Read the model definition and answer for the solid it produces. Units are mm, in the model's axes. A direction names the side the tool comes from. Coordinates: 2 decimals unless noted, no trailing zeros. Order: outer loops, then holes, each group sorted by start corner. A loop starts at its lowest first (then second) coordinate and runs counter-clockwise, first axis right, second up. Notation, with made-up numbers: (16, 17.5) -> (52, 17.5) arc R22 cw to (52, 34.5) -> close; hole circle Ø4 at (74, 6). An arc over 180 degrees is marked (long way). Answer as a JSON object with one key per item and string values. Group by question number.
1) Determine the mould class of faces 1 (the cylindrical face through (-6.17, 1.48, 4.68)), 2 (the cylindrical face through (0.931, 7.93, 2.957)), 3 (the flat face through (1.1, 13, -3.1)), 4 (the cylindrical face through (1.352, 7.93, 4.292)) for opening direction X: released by +X, released by -X, zero draft, split by the parting line, or undercut.
2) Section C-C on x = 0 is taken. Determine the outline of the cut face in (y, z).
3) Given pin 1 (4 mm diameter, centred on x = 4.95, z = 4.95, fed in from +Y); pin 2 (1 mm diameter, centred on x = 2.5, y = 9, fed in from +Z); pin 3 (4 mm diameter, centred on x = 4.5, y = 6.5, fed in from +Z); pin 4 (2 mm diameter, centred on x = 4.95, z = -4.95, fed in from +Y), each flat-ended and moving along its own axis, determine where each tip first touches the part or whether it passes through.
4) Consider L1, parallel to X at y = 2.25, z = 4.5; L2, parallel to Z at x = -5, y = 0.5; L3, parallel to X at y = 1.5, z = 5.5. Determine where each line is inside the solid, lowest interval first.
5) Section B-B on y = 8 is taken. Determine the outline of the cut face in (x, z).
6) Section D-D on y = 4.5 is taken. Determine the outline of the cut face in (x, z).
7) Section A-A on z = 0 is taken. Determine the outline of the cut face in (x, y), and give its area (3 significant figures).
8) A tool of negligible diameter and unlimited length cuts with its end or side. For faces 5 (the cylindrical face through (3.57, 7.39, -1.48)), 6 (the flat face through (-5, 3, 0)), from which of +Z, -Z, +X, -X, +Y, -Y can it reach the whole face along a straight path? Write none if from no direction.
from build123d import *

# Parameters (mm, degrees)
CROQUIS1_R                 = 12.5
CROQUIS1_R_2               = 1.25
SALIENTE_EXTRUIR1_DEPTH    = 3
SALIENTE_EXTRUIR2_START    = 3
CROQUIS1_3_R               = 4.5
CROQUIS1_3_R_2             = 3.1
SALIENTE_EXTRUIR2_DEPTH    = 10
CORTAR_EXTRUIR1_DEPTH      = 22.943108257
CORTAR_EXTRUIR1_DEPTH_BACK = 22.943108257
CROQUIS2_R                 = 1.6


with BuildPart() as part:
    # Croquis1 → Saliente-Extruir1 (new body)
    with BuildSketch(Plane(origin=(0, 0, 0), x_dir=(1, 0, 0), z_dir=(0, 1, 0))):
        with Locations(Location((0, 0, 0), (0, 0, 270))):
            Circle(CROQUIS1_R)
        with Locations(Location((-4.949747468, 4.949747468, 0), (0, 0, 270))):
            Circle(CROQUIS1_R_2, mode=Mode.SUBTRACT)
        with Locations(Location((4.949747468, 4.949747468, 0), (0, 0, 270))):
            Circle(CROQUIS1_R_2, mode=Mode.SUBTRACT)
        with Locations(Location((4.949747468, -4.949747468, 0), (0, 0, 270))):
            Circle(CROQUIS1_R_2, mode=Mode.SUBTRACT)
        with Locations(Location((-4.949747468, -4.949747468, 0), (0, 0, 270))):
            Circle(CROQUIS1_R_2, mode=Mode.SUBTRACT)
    extrude(amount=SALIENTE_EXTRUIR1_DEPTH)

    # Croquis1<3> → Saliente-Extruir2 (add)
    with BuildSketch(Plane(origin=(0, 0, 0), x_dir=(1, 0, 0), z_dir=(0, 1, 0)).offset(SALIENTE_EXTRUIR2_START)):
        with Locations(Location((0, 0, 0), (0, 0, 270))):
            Circle(CROQUIS1_3_R)
        with Locations(Location((0, 0, 0), (0, 0, 270))):
            Circle(CROQUIS1_3_R_2, mode=Mode.SUBTRACT)
    extrude(amount=SALIENTE_EXTRUIR2_DEPTH)

    # Croquis2 → Cortar-Extruir1 (cut, two sides: drawn at the far end of the back side and taken through both)
    with BuildSketch(Plane(origin=(0, 0, 0), x_dir=(0, 0, -1), z_dir=(1, 0, 0)).offset(-CORTAR_EXTRUIR1_DEPTH_BACK)):
        with Locations((0, 8)):
            Circle(CROQUIS2_R)
    extrude(amount=CORTAR_EXTRUIR1_DEPTH + CORTAR_EXTRUIR1_DEPTH_BACK, mode=Mode.SUBTRACT)


solid = part.part
Worked answers:
{
 "1": {"face 1": "undercut", "face 2": "undercut", "face 3": "zero draft", "face 4": "split by the parting line"},
 "2": {"outline": "(0, -12.5) -> (3, -12.5) -> (3, -4.5) -> (13, -4.5) -> (13, -3.1) -> (3, -3.1) -> (3, 3.1) -> (13, 3.1) -> (13, 4.5) -> (3, 4.5) -> (3, 12.5) -> (0, 12.5) -> close"},
 "3": {"pin 1": "stops at y = 3", "pin 2": "stops at z = 4.03", "pin 3": "stops at z = 3.74", "pin 4": "passes through"},
 "4": {"L1": "x = -11.66 to -6.12, -3.78 to 3.78, 6.12 to 11.66", "L2": "z = -11.46 to -6.2, -3.7 to 3.7, 6.2 to 11.46", "L3": "x = -11.22 to -6.07, -3.83 to 3.83, 6.07 to 11.22"},
 "5": {"outline": "(-4.21, -1.6) arc R4.5 ccw to (4.21, -1.6) -> (2.66, -1.6) arc R3.1 cw to (-2.66, -1.6) -> close; (-4.21, 1.6) -> (-2.66, 1.6) arc R3.1 cw to (2.66, 1.6) -> (4.21, 1.6) arc R4.5 ccw to start"},
 "6": {"outline": "circle Ø9 at (0, 0); hole circle Ø6.2 at (0, 0)"},
 "7": {"outline": "(-12.5, 0) -> (12.5, 0) -> (12.5, 3) -> (4.5, 3) -> (4.5, 6.4) -> (3.1, 6.4) -> (3.1, 3) -> (-3.1, 3) -> (-3.1, 6.4) -> (-4.5, 6.4) -> (-4.5, 3) -> (-12.5, 3) -> close; (-4.5, 9.6) -> (-3.1, 9.6) -> (-3.1, 13) -> (-4.5, 13) -> close; (3.1, 9.6) -> (4.5, 9.6) -> (4.5, 13) -> (3.1, 13) -> close", "area": "94.0 mm²"},
 "8": {"face 5": "+X, -X", "face 6": "+Y"}
}
